The drawing under review shows one solid part. Ordinate dimensions are in mm from its lowest x, y, z. A direction names the side the tool comes from. Give positions to 0.01 mm unless a question says otherwise; leave off trailing zeros. Loops run counter-clockwise (first coordinate to the right, second up) from the corner with the lowest first, then second, coordinate; pieces in that order, holes last. Notation, with made-up numbers: (49, 22.5) -> (95, 22.5) arc R31 ccw to (95, 55.5) -> close; hole circle Ø4 at (-23, 43.25). An arc over 180 degrees is marked (long way). Answer in a Markdown table with one row per item. Add a question column.
(1) For the marked faces 4 and 5, list the 3-axis set-ups (+Z, -Z, +X, -X, +Y, -Y) from which the entire face can be reached by the end or side of a thin tool; tool diameter is ignored.
(2) For line 1 (Y direction, x = 6, z = 12.4); line 2 (Y direction, x = 6, z = 4.5); line 3 (Z direction, x = 3, y = 28), list the stretches that pass through material, from the lowest coordinate up.
(3) Draft analysis for pull direction Y (two halves, no side actions). For the marked faces 1, 2 and 3, state which applies: +Y half, -Y half, draft (parallel to the pull), parting line (faces both ways), or undercut.
(4) Consider section C-C on y = 15. Write out the cut boundary in (x, z), then the cut area to 3 significant figures.
(5) Consider section D-D on y = 4.25. Write out the cut boundary in (x, z).
(6) Consider section B-B on z = 11. Write out the cut boundary in (x, y), then the cut area to 3 significant figures.
(7) Consider section A-A on x = 6. Write out the cut boundary in (y, z), then the cut area to 3 significant figures.
(8) For pin 1 (3.5 mm diameter, centred on x = 6, y = 5, fed in from +Z); pin 2 (3 mm diameter, centred on x = 1.5, y = 12, fed in from -Z); pin 3 (5 mm diameter, centred on x = 2, y = 11, fed in from -Z); pin 4 (1.5 mm diameter, centred on x = 2, z = 2.5, fed in from -Y), all flat-tipped, find the tip position at first contact; note any pin that passes through.
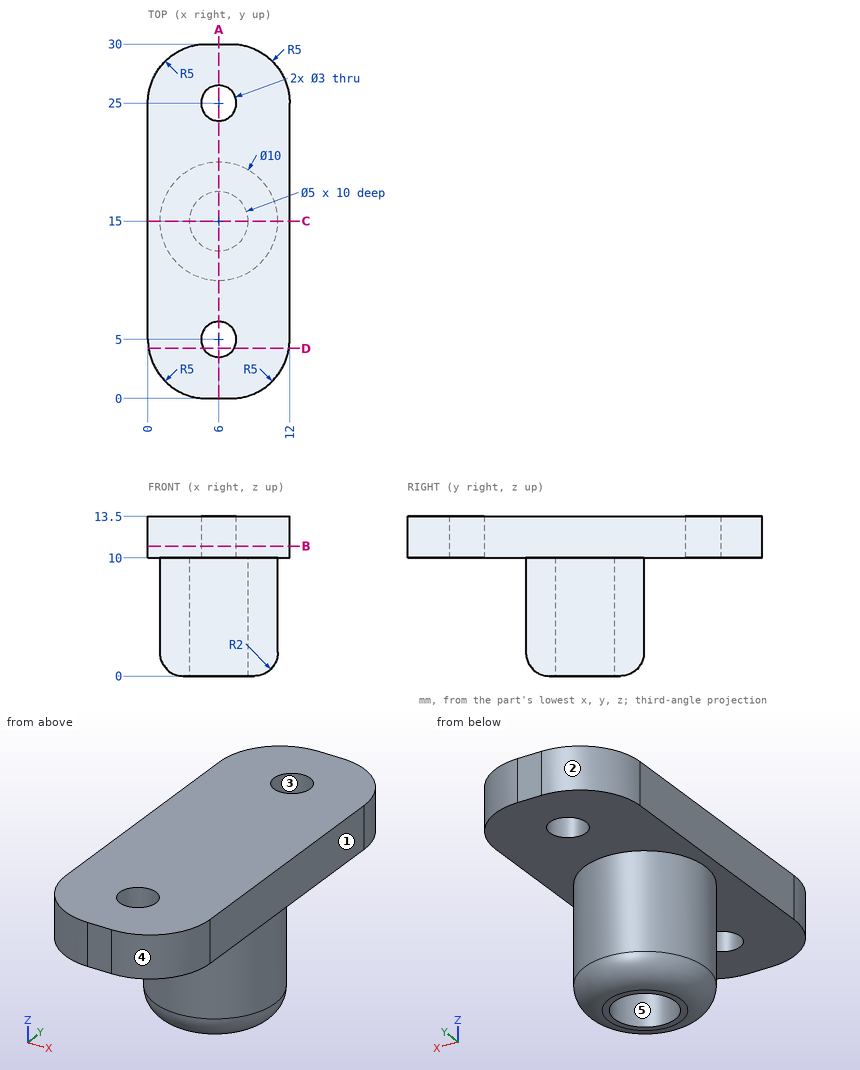
Values follow:
| question | item | result |
|---|---|---|
| 1 | face 4 | +Z, -Z, +X, -Y |
| 1 | face 5 | -Z |
| 2 | line 1 | 0 to 3.5, 6.5 to 23.5, 26.5 to 30 |
| 2 | line 2 | 10 to 12.5, 17.5 to 20 |
| 2 | line 3 | 10 to 13.5 |
| 3 | face 1 | draft |
| 3 | face 2 | +Y half |
| 3 | face 3 | undercut |
| 4 | outline | (0, 10) -> (1, 10) -> (1, 2) arc R2 ccw to (3, 0) -> (3.5, 0) -> (3.5, 10) -> (8.5, 10) -> (8.5, 0) -> (9, 0) arc R2 ccw to (11, 2) -> (11, 10) -> (12, 10) -> (12, 13.5) -> (0, 13.5) -> close |
| 4 | area | 90.3 mm2 |
| 5 | outline | (0.06, 10) -> (4.7, 10) -> (4.7, 13.5) -> (0.06, 13.5) -> close; (7.3, 10) -> (11.94, 10) -> (11.94, 13.5) -> (7.3, 13.5) -> close |
| 6 | outline | (0, 5) arc R5 ccw to (5, 0) -> (7, 0) arc R5 ccw to (12, 5) -> (12, 25) arc R5 ccw to (7, 30) -> (5, 30) arc R5 ccw to (0, 25) -> close; hole circle Ø3 at (6, 5); hole circle Ø3 at (6, 25) |
| 6 | area | 324 mm2 |
| 7 | outline | (0, 10) -> (3.5, 10) -> (3.5, 13.5) -> (0, 13.5) -> close; (6.5, 10) -> (10, 10) -> (10, 2) arc R2 ccw to (12, 0) -> (12.5, 0) -> (12.5, 10) -> (17.5, 10) -> (17.5, 0) -> (18, 0) arc R2 ccw to (20, 2) -> (20, 10) -> (23.5, 10) -> (23.5, 13.5) -> (6.5, 13.5) -> close; (26.5, 10) -> (30, 10) -> (30, 13.5) -> (26.5, 13.5) -> close |
| 7 | area | 132 mm2 |
| 8 | pin 1 | z = 13.5 |
| 8 | pin 2 | z = 0.22 |
| 8 | pin 3 | z = 0.01 |
| 8 | pin 4 | y = 11.2 |
